from build123d import *

# Parameters (mm, degrees)
F0_W     = 89
F0_H     = 45
F0_R     = 2.5
F0_W_2   = 3
F1_DEPTH = 1.6
F2_DEPTH = 6
F3_W     = 6
F3_H     = 6
F3_W_2   = 83
F3_H_2   = 33
F4_DEPTH = 3
F5_W     = 28.891159
F5_H     = 28.9066
F5_W_2   = 21.864466
F5_H_2   = 21.864466
F6_DEPTH = 2
F7_R     = 0.6
F8_DEPTH = 6
F9_SIZE  = 2.2


with BuildPart() as f1:
    # F0 (on Top) → F1 (new body)
    with BuildSketch(Plane.XY):
        Rectangle(F0_W, F0_H)
        with Locations((-12.7, -12.7)):
            Circle(F0_R, mode=Mode.SUBTRACT)
        with Locations((12.7, -12.7)):
            Circle(F0_R, mode=Mode.SUBTRACT)
        with Locations((-12.7, 12.7)):
            Circle(F0_R, mode=Mode.SUBTRACT)
        with Locations((12.7, 12.7)):
            Circle(F0_R, mode=Mode.SUBTRACT)
        with Locations((46, 0)):
            Rectangle(F0_W_2, F0_H)
        with Locations((-46, 0)):
            Rectangle(F0_W_2, F0_H)
        with Locations((-12.7, 12.7)):
            Circle(F0_R)
        with Locations((12.7, 12.7)):
            Circle(F0_R)
        with Locations((12.7, -12.7)):
            Circle(F0_R)
        with Locations((-12.7, -12.7)):
            Circle(F0_R)
    extrude(amount=F1_DEPTH)

    # F0 (on Top) → F2 (join)
    with BuildSketch(Plane.XY):
        with Locations((-12.7, -12.7)):
            Circle(F0_R)
        with Locations((-12.7, 12.7)):
            Circle(F0_R)
        with Locations((12.7, -12.7)):
            Circle(F0_R)
        with Locations((12.7, 12.7)):
            Circle(F0_R)
    extrude(amount=F2_DEPTH)

    # F3 (on face) → F4 (join)
    with BuildSketch(Plane.XY.offset(1.6)):
        with Locations((-44.5, 19.5)):
            Rectangle(F3_W, F3_H)
        with Locations((0, 19.5)):
            Rectangle(F3_W_2, F3_H)
        with Locations((-44.5, 0)):
            Rectangle(F3_W, F3_H_2)
        with Locations((44.5, 19.5)):
            Rectangle(F3_W, F3_H)
        with Locations((-44.5, -19.5)):
            Rectangle(F3_W, F3_H)
        with Locations((44.5, 0)):
            Rectangle(F3_W, F3_H_2)
        with Locations((0, -19.5)):
            Rectangle(F3_W_2, F3_H)
        with Locations((44.5, -19.5)):
            Rectangle(F3_W, F3_H)
    extrude(amount=F4_DEPTH)

    # F5 (on face) → F6 (join)
    with BuildSketch(Plane.XY.offset(1.6)):
        with Locations((-0.254421, -0.2533)):
            Rectangle(F5_W, F5_H)
        Rectangle(F5_W_2, F5_H_2, mode=Mode.SUBTRACT)
    extrude(amount=F6_DEPTH)

    # F7 (on face) → F8 (cut)
    with BuildSketch(Plane.XY.offset(6)):
        with Locations((-12.7, 12.7)):
            Circle(F7_R)
        with Locations((12.7, 12.7)):
            Circle(F7_R)
        with Locations((12.7, -12.7)):
            Circle(F7_R)
        with Locations((-12.7, -12.7)):
            Circle(F7_R)
    extrude(amount=-F8_DEPTH, mode=Mode.SUBTRACT)

    # F9
    f9_edges = [f1.edges().sort_by_distance(p)[0] for p in [
        (0, 16.5, 4.6),
        (-41.5, 0, 4.6),
        (-47.5, 0, 4.6),
        (0, 22.5, 4.6),
        (0, -22.5, 4.6),
        (47.5, 0, 4.6),
        (41.5, 0, 4.6),
        (0, -16.5, 4.6),
    ]]
    chamfer(f9_edges, length=F9_SIZE)


solid = f1.part
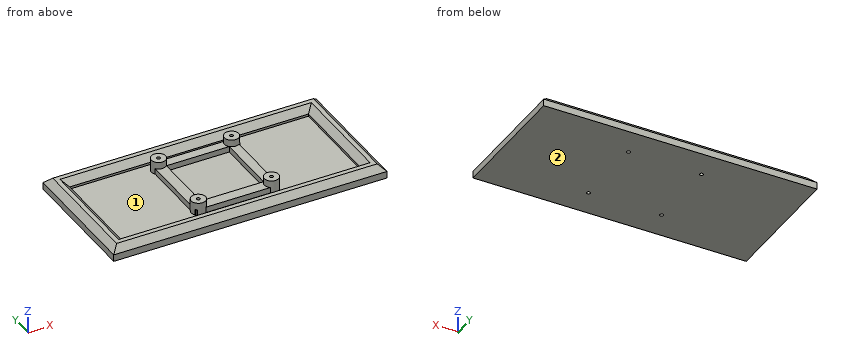
For this review, take the finished solid that the model builds, in its own axes (mm). Face numbers are marked on the shaded views. Give positions to 0.01 mm unless a question says otherwise; leave off trailing zeros. Write each loop counter-clockwise with the first axis right and the second up, starting at its lowest first coordinate (ties: lowest second). Pieces come first, ordered by that corner, then holes. Notation, with made-up numbers: (85, 83.5) -> (143, 83.5) arc R31 cw to (143, 113.5) -> close; hole circle Ø3 at (-36, 33.25). An arc over 180 degrees is marked (long way). Use CSV: the item, a comma, the result in double quotes.
Q1. Take a section at A-A, the plane x = -33.5. Write out the cut boundary in (y, z), then the cut area to 3 significant figures.
Conclusion:
outline,"(-22.5, 0) -> (22.5, 0) -> (22.5, 2.4) -> (20.3, 4.6) -> (18.7, 4.6) -> (16.5, 2.4) -> (16.5, 1.6) -> (-16.5, 1.6) -> (-16.5, 2.4) -> (-18.7, 4.6) -> (-20.3, 4.6) -> (-22.5, 2.4) -> close"
area,"98.3 mm2"
Q2. For P1, Ø1, axis at x = 12.5, y = -5, coming from the +Z side; P2, Ø1, axis at y = -15.5, z = 5, coming from the +X side; P3, Ø1.5, axis at x = 22.5, z = 5, coming from the -Y side, all flat-tipped, find the tip position at first contact; note any pin that passes through.
Conclusion:
P1,"z = 3.6"
P2,"x = 45.4"
P3,"y = -20.65"
Q3. To check wall thickness, follow probe 1 along Y at (x, z) = (12.7, 4.3); probe 2 along Y at (x, z) = (26.5, 2.2); probe 3 along Z at (x, y) = (-19, 0). State the ranges of each line that lie inside material, in increasing order. Write a range as [from, to].
Conclusion:
probe 1,"[-20.6, -18.4], [-15.2, -13.3], [-12.1, -10.2], [10.2, 12.1], [13.3, 15.2], [18.4, 20.6]"
probe 2,"[-22.5, -16.5], [16.5, 22.5]"
probe 3,"[0, 1.6]"
Q4. Mouldability with a two-part tool opening along Y and no side actions: class the marked faces 1 and 2 as pulls with the +Y half, pulls with the -Y half, needs draft (parallel to the pull), parting line crosses it, or undercut.
Conclusion:
face 1,"undercut"
face 2,"needs draft"
Q5. Take a section at B-B, the plane x = -4. Write out the cut boundary in (y, z).
Conclusion:
outline,"(-22.5, 0) -> (22.5, 0) -> (22.5, 2.4) -> (20.3, 4.6) -> (18.7, 4.6) -> (16.5, 2.4) -> (16.5, 1.6) -> (14.2, 1.6) -> (14.2, 3.6) -> (10.93, 3.6) -> (10.93, 1.6) -> (-10.93, 1.6) -> (-10.93, 3.6) -> (-14.71, 3.6) -> (-14.71, 1.6) -> (-16.5, 1.6) -> (-16.5, 2.4) -> (-18.7, 4.6) -> (-20.3, 4.6) -> (-22.5, 2.4) -> close"
